Check sheet for the modelled part. Datum: model origin and axes. Units: mm. Face numbers are marked on the shaded views. A direction names the side the tool comes from. Give positions to 0.01 mm unless a question says otherwise; leave off trailing zeros. Order: outer loops, then holes, each group sorted by start corner. A loop starts at its lowest first (then second) coordinate and runs counter-clockwise, first axis right, second up.
Autodesk Inventor part; units mm, degrees
ref_plane "to_bolt_XY" through (4, -6, 0) normal (1, 0, 0) x (0, 0, -1)
ref_plane "to_bolt_YZ" through (4, -6, 0) normal (0, 0, -1) x (0, 1, 0)
ref_plane "to_bolt_ZX" through (4, -6, 0) normal (0, 1, 0) x (1, 0, 0)
sketch "Sketch_14" plane through (0, 0, 0) normal (1, 0, 0) x (0, 1, 0)
  line L0 (0, -4) -> (0, 4)
  line L1 (0, 4) -> (9.5, 4)
  line L2 (9.5, 4) -> (10, 3.5)
  line L3 (10, 3.5) -> (10, -3.5)
  line L4 (10, -3.5) -> (9.5, -4)
  line L5 (9.5, -4) -> (0, -4)
  line L6 (0, -4) -> (0, 4)
revolve "Revolution1" add sketch "Sketch_14" angle 360 about axis through (0, 0, -4) along (0, 0, -1)
sketch "Sketch_15" plane through (0, 0, 0) normal (1, 0, 0) x (0, 1, 0)
  line L0 (0, -4) -> (0, 4)
  line L1 (0, 4) -> (3.5, 4)
  line L2 (3.5, 4) -> (3, 3.5)
  line L3 (3, 3.5) -> (3, -3.5)
  line L4 (3, -3.5) -> (3.5, -4)
  line L5 (3.5, -4) -> (0, -4)
  line L6 (0, -4) -> (0, 4)
revolve "Revolution2" cut sketch "Sketch_15" angle 360 about axis through (0, 0, -4) along (0, 0, -1)
sketch "Sketch_16" plane through (0, 0, 0) normal (0, 0, 1) x (1, 0, 0)
  arc A0 (-0.5, -10.9886) -> (0.5, -10.9886) centre (0, 0) ccw
  line L0 (0.5, -10.9886) -> (0.5, 0)
  line L1 (0.5, 0) -> (-0.5, 0)
  line L2 (-0.5, 0) -> (-0.5, -10.9886)
extrude "Extrusion1" cut sketch "Sketch_16" along normal mid plane 8
sketch "Sketch4" plane through (0, 0, -4) normal (0, 0, -1) x (-1, 0, 0)
  point P0 (-6, 0)
hole "Hole1" at (6, 0, -4) direction (0, 0, 1) diameter 3.5 depth 8
sketch "Sketch5" plane through (0, 0, -4) normal (0, 0, -1) x (-1, 0, 0)
  point P0 (6, 0)
hole "Hole2" at (-6, 0, -4) direction (0, 0, 1) diameter 3.5 depth 8
sketch "Sketch6" plane through (0, 0, -4) normal (0, 0, -1) x (-1, 0, 0)
  point P0 (0, 6)
hole "Hole3" at (0, 6, -4) direction (0, 0, 1) diameter 3.5 depth 8
sketch "Sketch_23" plane through (0, -6, 0) normal (0, 1, 0) x (1, 0, 0)
  line L0 (10, 0) -> (0, 0)
  line L1 (0, 0) -> (0, 1.7)
  line L2 (0, 1.7) -> (4, 1.7)
  line L3 (4, 1.7) -> (4, 3)
  line L4 (4, 3) -> (10, 3)
  line L5 (10, 3) -> (10, 0)
  line L6 (10, 0) -> (0, 0)
revolve "Revolution3" cut sketch "Sketch_23" angle 360 about axis through (10, -6, 0) along (1, 0, 0)
sketch "Sketch8" plane through (-0.5, -9.4868, 4) normal (1, 0, 0) x (0, 0, -1)
  point P0 (4, 3.4868)
hole "Hole4" at (-0.5, -6, 0) direction (-1, 0, 0) diameter 2.459 depth 8.4303 countersink diameter 3 countersink angle 90
ref_plane "to_bolt_XY" through (4, -6, 0) normal (1, 0, 0) x (0, 0, -1)
ref_plane "to_bolt_YZ" through (4, -6, 0) normal (0, 0, -1) x (0, 1, 0)
ref_plane "to_bolt_ZX" through (4, -6, 0) normal (0, 1, 0) x (1, 0, 0)
properties part number "SCST6-8b"
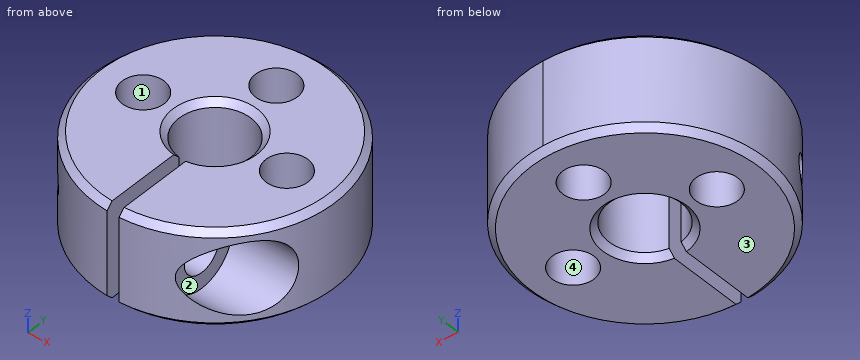
(1) Release check for a two-part mould opening along Y. For the marked faces 3 and 4 record: released by +Y, released by -Y, zero draft, split by the parting line, or undercut.
Response values:
face 3: zero draft
face 4: undercut
(2) Material ranges on L1, parallel to X at y = 0, z = -1; L2, parallel to Y at x = -0.75, z = -1; L3, parallel to Y at x = -6.5, z = 0, recorded low to high.
Response values:
L1: x = -10 to -7.75, -4.25 to -3, 3 to 4.25, 7.75 to 10
L2: y = -9.97 to -6.75, -5.25 to -2.9, 2.9 to 4.42, 7.58 to 9.97
L3: y = -7.6 to -7.23, -4.77 to -1.68, 1.68 to 7.6
(3) Set-up check for the marked faces 1 and 2: record each of +Z, -Z, +X, -X, +Y, -Y from which the full face is reachable in a straight line by a thin tool's end or side.
Response values:
face 1: +Z, -Z
face 2: +X
(4) Cross-section at D-D on x = 0.75. Count the separate pieces of the cut face and the enclosed holes in it, then the cut area to 3 significant figures.
Response values:
separate pieces: 3
enclosed holes: 1
area: 77.7 mm2
(5) Cross-section at C-C on z = 3.25. Enter the section's corners in (x, y), then the cut area to 3 significant figures.
Response values:
outline: (-0.5, -9.99) - (-0.5, -2.96) arc R3 cw (long way) to (0.5, -2.96) - (0.5, -9.99) arc R10 ccw (long way) to start; hole circle Ø3.5 at (-6, 0); hole circle Ø3.5 at (0, 6); hole circle Ø3.5 at (6, 0)
area: 250 mm2
(6) Cross-section at A-A on z = 0. Enter the section's corners in (x, y), then the cut area to 3 significant figures.
Response values:
outline: (-8.79, -4.77) - (-0.77, -4.77) - (-0.5, -4.5) - (-0.5, -2.96) arc R3 cw (long way) to (0.5, -2.96) - (0.5, -4.3) - (4, -4.3) - (4, -3) - (9.54, -3) arc R10 ccw (long way) to start; (-6.91, -7.23) arc R10 ccw to (-0.5, -9.99) - (-0.5, -7.5) - (-0.77, -7.23) - close; (0.5, -9.99) arc R10 ccw to (4.36, -9) - (4, -9) - (4, -7.7) - (0.5, -7.7) - close; hole circle Ø3.5 at (-6, 0); hole circle Ø3.5 at (0, 6); hole circle Ø3.5 at (6, 0)
area: 198 mm2
(7) Gauge pin test, flat ends, axial feed: pin 1 Ø1.5 at (x, z) = (3, 2.5) entering from +Y; pin 2 Ø3 at (y, z) = (6.5, -0.5) entering from -X; pin 3 Ø2 at (y, z) = (-2.5, 0) entering from -X. Record the tip position at first contact, or that the pin passes through.
Response values:
pin 1: stops at y = 9.74
pin 2: stops at x = -8.66
pin 3: stops at x = -9.89
(8) Cross-section at B-B on y = 0. Enter the section's corners in (x, z).
Response values:
outline: (-10, -3.5) - (-9.5, -4) - (-7.75, -4) - (-7.75, 4) - (-9.5, 4) - (-10, 3.5) - close; (-4.25, -4) - (-3.5, -4) - (-3, -3.5) - (-3, 3.5) - (-3.5, 4) - (-4.25, 4) - close; (3, -3.5) - (3.5, -4) - (4.25, -4) - (4.25, 4) - (3.5, 4) - (3, 3.5) - close; (7.75, -4) - (9.5, -4) - (10, -3.5) - (10, 3.5) - (9.5, 4) - (7.75, 4) - close
